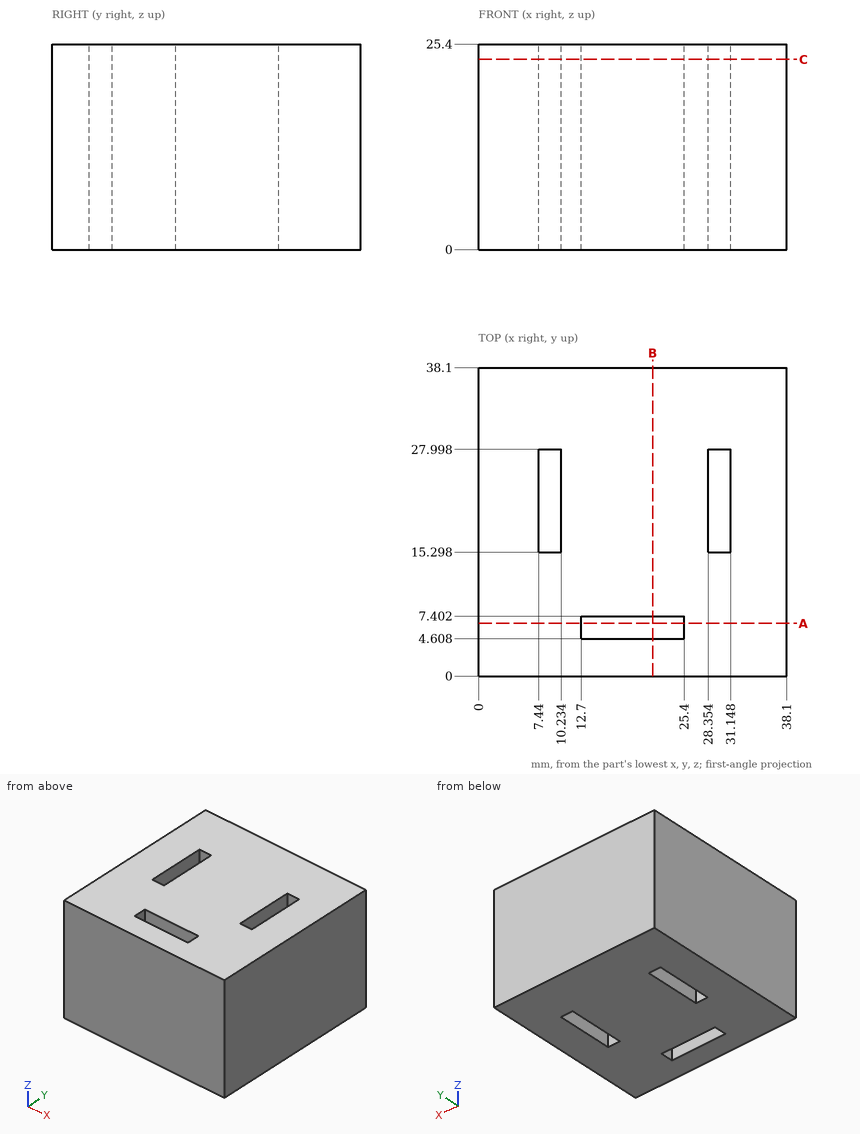
Source: three-view drawing plus pictorial views. Frame: mm from the lowest corner of the part. Round coordinates to 2 decimals unless told otherwise and drop trailing zeros. Loops run counter-clockwise (first coordinate to the right, second up) from the corner with the lowest first, then second, coordinate; pieces in that order, holes last. Notation, with made-up numbers: (82.5, -33) -> (126.5, -33) arc R16 ccw to (126.5, -6) -> close; hole circle Ø1 at (-27.5, 84.25). An arc over 180 degrees is marked (long way). Use one line per item in the form item = value.
Item 1: Cut plane C-C on z = 23.5. Output: boundary loops of the cut face in (x, y), then the cut area to 3 significant figures.
Evaluation:
outline = (0, 0) -> (38.1, 0) -> (38.1, 38.1) -> (0, 38.1) -> close; hole (7.44, 15.3) -> (10.23, 15.3) -> (10.23, 28) -> (7.44, 28) -> close; hole (12.7, 4.61) -> (25.4, 4.61) -> (25.4, 7.4) -> (12.7, 7.4) -> close; hole (28.35, 15.3) -> (31.15, 15.3) -> (31.15, 28) -> (28.35, 28) -> close
area = 1,350 mm2
Item 2: Cut plane A-A on y = 6.5. Output: boundary loops of the cut face in (x, z).
Evaluation:
outline = (0, 0) -> (12.7, 0) -> (12.7, 25.4) -> (0, 25.4) -> close; (25.4, 0) -> (38.1, 0) -> (38.1, 25.4) -> (25.4, 25.4) -> close
Item 3: Cut plane B-B on x = 21.5. Output: boundary loops of the cut face in (y, z).
Evaluation:
outline = (0, 0) -> (4.61, 0) -> (4.61, 25.4) -> (0, 25.4) -> close; (7.4, 0) -> (38.1, 0) -> (38.1, 25.4) -> (7.4, 25.4) -> close
Item 4: Material intervals for probe 1 along X at (y, z) = (21, 13.25); probe 2 along Y at (x, z) = (19, 15.25), sorted ascending.
Evaluation:
probe_1 = 0 to 7.44, 10.23 to 28.35, 31.15 to 38.1
probe_2 = 0 to 4.61, 7.4 to 38.1
